The model under review builds one solid part; all positions refer to its coordinate system, in mm. Face numbers are marked on the shaded views. Coordinates: 2 decimals unless noted, no trailing zeros. Loops run counter-clockwise (first coordinate to the right, second up) from the corner with the lowest first, then second, coordinate; pieces in that order, holes last. Notation, with made-up numbers: (-12, 25.5) - (13, 25.5) arc R28 cw to (13, 48.5) - close; hole circle Ø2 at (22.25, 43.5). An arc over 180 degrees is marked (long way). Answer in a Markdown table with one row per item. Add a question column.
(1) We need section C-C on z = -4. Give the number of separate pieces and of enclosed holes in the cut face, plus the area to 3 significant figures.
(2) We need section B-B on y = 19.5. Write out the cut boundary in (x, z).
(3) We need section A-A on x = 29. Write out the cut boundary in (y, z), plus the area to 3 significant figures.
(4) For P1, Ø4, axis at x = 20, y = 20.5, coming from the +Z side; P2, Ø0.5, axis at x = 18, y = 32, coming from the -Z side; P3, Ø4, axis at x = 26, y = 20, coming from the -Z side; P4, Ø1.3, axis at x = 4, y = 4, coming from the -Z side, all flat-tipped, find the tip position at first contact; note any pin that passes through.
(5) Mouldability with a two-part tool opening along Y and no side actions: class the marked faces 1 and 2 as +Y half, -Y half, draft (parallel to the pull), parting line (faces both ways), or undercut.
(6) We need section D-D on y = 4. Write out the cut boundary in (x, z).
(7) For line 1 along X through (y, z) = (4, -2.35); line 2 along Y through (x, z) = (4, -3.65); line 3 along Y through (x, z) = (25.5, 2.5), list the stretches that pass through material, from the lowest coordinate up.
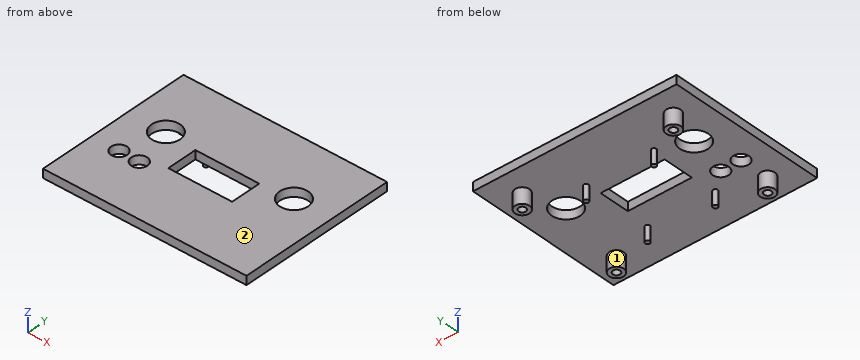
from build123d import *

# Parameters (mm, degrees)
SZKIC1_W                    = 70.000011125
SZKIC1_H                    = 54.450044047
SZKIC1_R                    = 4.901215244
SZKIC1_R_2                  = 2.75
SZKIC1_W_2                  = 22
SZKIC1_H_2                  = 10.5
DODANIE_WYCI_GNI_CIE2_DEPTH = 3
SZKIC3_R                    = 2.5
DODANIE_WYCI_GNI_CIE3_DEPTH = 5.3
SZKIC5_R                    = 1.25
WYTNIJ_WYCI_GNI_CIE1_DEPTH  = 5
SZKIC6_R                    = 0.8
DODANIE_WYCI_GNI_CIE4_DEPTH = 5


with BuildPart() as part:
    # Szkic1 → Dodanie-wyciągnięcie2 (new body)
    with BuildSketch(Plane.XY):
        with Locations((29.999994437, 22.225000357)):
            Rectangle(SZKIC1_W, SZKIC1_H)
        with Locations((8.033600802, 27.9335383)):
            Circle(SZKIC1_R, mode=Mode.SUBTRACT)
        with Locations((51.966399076, 28.066461662)):
            Circle(SZKIC1_R, mode=Mode.SUBTRACT)
        with Locations((4.47500206, 13.790057549)):
            Circle(SZKIC1_R_2, mode=Mode.SUBTRACT)
        with Locations((11.475021134, 13.75003756)):
            Circle(SZKIC1_R_2, mode=Mode.SUBTRACT)
        with Locations((29.933998796, 21.819981485)):
            Rectangle(SZKIC1_W_2, SZKIC1_H_2, mode=Mode.SUBTRACT)
    extrude(amount=DODANIE_WYCI_GNI_CIE2_DEPTH)

    # Szkic3 → Dodanie-wyciągnięcie3 (add)
    with BuildSketch(Plane(origin=(0, 0, 0), x_dir=(-1, 0, 0), z_dir=(0, 0, -1))):
        with Locations((-55.99999976, 40.50000028)):
            Circle(SZKIC3_R)
        with Locations((-3.99999962, 40.50000028)):
            Circle(SZKIC3_R)
        with Locations((-55.99999976, 3.99999962)):
            Circle(SZKIC3_R)
        with Locations((-3.99999962, 3.99999962)):
            Circle(SZKIC3_R)
    extrude(amount=DODANIE_WYCI_GNI_CIE3_DEPTH)

    # Szkic5 → Wytnij-wyciągnięcie1 (cut)
    with BuildSketch(Plane(origin=(0, 0, -5.3), x_dir=(-1, 0, 0), z_dir=(0, 0, -1))):
        with Locations((-55.99999976, 40.50000028)):
            Circle(SZKIC5_R)
        with Locations((-3.99999962, 40.50000028)):
            Circle(SZKIC5_R)
        with Locations((-55.99999976, 3.99999962)):
            Circle(SZKIC5_R)
        with Locations((-3.99999962, 3.99999962)):
            Circle(SZKIC5_R)
    extrude(amount=-WYTNIJ_WYCI_GNI_CIE1_DEPTH, mode=Mode.SUBTRACT)

    # Szkic6 → Dodanie-wyciągnięcie4 (add)
    with BuildSketch(Plane(origin=(0, 0, 0), x_dir=(-1, 0, 0), z_dir=(0, 0, -1))):
        with Locations((-41.583998796, 31.969981485)):
            Circle(SZKIC6_R)
        with Locations((-18.283998796, 31.969981485)):
            Circle(SZKIC6_R)
        with Locations((-41.583998796, 8.169981485)):
            Circle(SZKIC6_R)
        with Locations((-18.283998796, 8.169981485)):
            Circle(SZKIC6_R)
    extrude(amount=DODANIE_WYCI_GNI_CIE4_DEPTH)


solid = part.part
Outcome:
| question | item | result |
|---|---|---|
| 1 | separate pieces | 8 |
| 1 | enclosed holes | 4 |
| 1 | area | 66.9 mm² |
| 2 | outline | (-5, 0) - (18.93, 0) - (18.93, 3) - (-5, 3) - close; (40.93, 0) - (65, 0) - (65, 3) - (40.93, 3) - close |
| 3 | outline | (-5, 0) - (16.57, 0) - (16.57, 3) - (-5, 3) - close; (27.07, 0) - (49.45, 0) - (49.45, 3) - (27.07, 3) - close |
| 3 | area | 132 mm² |
| 4 | P1 | z = 3 |
| 4 | P2 | z = -5 |
| 4 | P3 | through |
| 4 | P4 | z = -0.3 |
| 5 | face 1 | undercut |
| 5 | face 2 | draft |
| 6 | outline | (-5, 0) - (1.5, 0) - (1.5, -5.3) - (2.75, -5.3) - (2.75, -0.3) - (5.25, -0.3) - (5.25, -5.3) - (6.5, -5.3) - (6.5, 0) - (53.5, 0) - (53.5, -5.3) - (54.75, -5.3) - (54.75, -0.3) - (57.25, -0.3) - (57.25, -5.3) - (58.5, -5.3) - (58.5, 0) - (65, 0) - (65, 3) - (-5, 3) - close |
| 7 | line 1 | 1.5 to 2.75, 5.25 to 6.5, 53.5 to 54.75, 57.25 to 58.5 |
| 7 | line 2 | 1.5 to 2.75, 5.25 to 6.5, 38 to 39.25, 41.75 to 43 |
| 7 | line 3 | -5 to 16.57, 27.07 to 49.45 |
